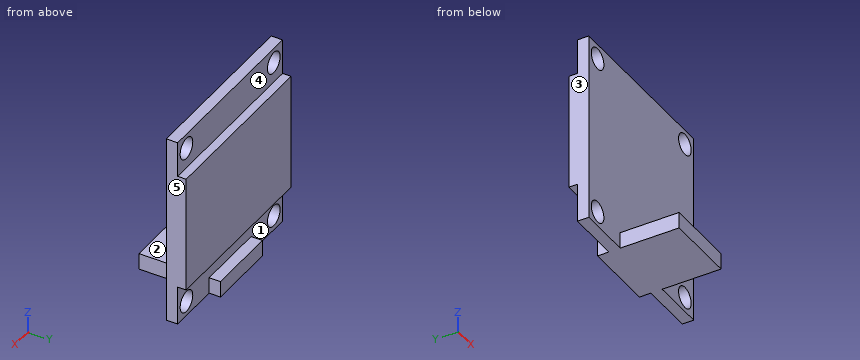
from build123d import *

# Parameters (mm, degrees)
SKETCH_1_W           = 25
SKETCH_1_H           = 27
EXTRUDE_1_DEPTH      = 1.6
SKETCH_2_W           = 25
SKETCH_2_H           = 16.5
EXTRUDE_2_DEPTH      = 1.2
SKETCH_3_R           = 1.5
CUT_EXTRUDE_1_DEPTH  = 37.83150825
EXTRUDE_4_DEPTH      = 1.6
EXTRUDE_4_DEPTH_BACK = 9.9
SKETCH_5_W           = 10
SKETCH_5_H           = 2.3


with BuildPart() as part:
    # 草图1 → 凸台-拉伸1 (new body)
    with BuildSketch(Plane(origin=(0, 0, 0), x_dir=(1, 0, 0), z_dir=(0, 1, 0))):
        with Locations((12.5, 13.5)):
            Rectangle(SKETCH_1_W, SKETCH_1_H)
    extrude(amount=EXTRUDE_1_DEPTH)

    # 草图2 → 凸台-拉伸2 (add)
    with BuildSketch(Plane(origin=(0, 1.6, 0), x_dir=(1, 0, 0), z_dir=(0, 1, 0))):
        with Locations((12.5, 13.25)):
            Rectangle(SKETCH_2_W, SKETCH_2_H)
    extrude(amount=EXTRUDE_2_DEPTH)

    # 草图3 → 切除-拉伸1 (cut, through all)
    with BuildSketch(Plane(origin=(0, 1.6, 0), x_dir=(1, 0, 0), z_dir=(0, 1, 0))):
        with Locations(Location((2.1, 24.9, 0), (0, 0, 270))):
            Circle(SKETCH_3_R)
        with Locations(Location((22.9, 24.9, 0), (0, 0, 90))):
            Circle(SKETCH_3_R)
        with Locations(Location((22.9, 2.1, 0), (0, 0, 270))):
            Circle(SKETCH_3_R)
        with Locations(Location((2.1, 2.1, 0), (0, 0, 90))):
            Circle(SKETCH_3_R)
    extrude(amount=-CUT_EXTRUDE_1_DEPTH, mode=Mode.SUBTRACT)

    # 草图5 → 凸台-拉伸4 (add, two sides: drawn at the far end of the back side and taken through both)
    with BuildSketch(Plane(origin=(0, 1.6, 0), x_dir=(1, 0, 0), z_dir=(0, 1, 0)).offset(-EXTRUDE_4_DEPTH_BACK)):
        with Locations((12.5, 25.85)):
            Rectangle(SKETCH_5_W, SKETCH_5_H)
    extrude(amount=EXTRUDE_4_DEPTH + EXTRUDE_4_DEPTH_BACK)


solid = part.part
Source: CAD feature listing. Evaluate the final solid. Frame: model axes, mm. Face numbers are marked on the shaded views. A direction names the side the tool comes from. Coordinates: 2 decimals unless noted, no trailing zeros. Write each loop counter-clockwise with the first axis right and the second up, starting at its lowest first coordinate (ties: lowest second). Pieces come first, ordered by that corner, then holes. Notation, with made-up numbers: M 72.5,26.25 L 127.5,26.25 A3 ccw 127.5,30.25 Z; hole C 55,55.25 d9. An arc over 180 degrees is marked long. Use a Markdown table: item, result.
1) Ray query, L1, parallel to X at y = 1.15, z = -2.1; L2, parallel to Z at x = 13.75, y = -7.5; L3, parallel to Y at x = 18.75, z = -12.75. Return the intervals inside material, ascending.
Conclusion:
| item | result |
|---|---|
| L1 | x = 0 to 0.6, 3.6 to 21.4, 24.4 to 25 |
| L2 | z = -27 to -24.7 |
| L3 | y = 0 to 2.8 |
2) Section C-C, the plane x = 5.5. Output: boundary loops of the cut face in (y, z).
Conclusion:
| item | result |
|---|---|
| outline | M 0,-27 L 1.6,-27 L 1.6,-21.5 L 2.8,-21.5 L 2.8,-5 L 1.6,-5 L 1.6,0 L 0,0 Z |
3) Section A-A, the plane z = -2.1. Output: boundary loops of the cut face in (x, y), then the cut area to 3 significant figures.
Conclusion:
| item | result |
|---|---|
| outline | M 0,0 L 0.6,0 L 0.6,1.6 L 0,1.6 Z; M 3.6,0 L 21.4,0 L 21.4,1.6 L 3.6,1.6 Z; M 24.4,0 L 25,0 L 25,1.6 L 24.4,1.6 Z |
| area | 30.4 mm^2 |
4) First-contact query: pin 1 Ø5 at (x, z) = (14.5, -10.5) entering from +Y; pin 2 Ø1.3 at (x, y) = (18, 2.5) entering from +Z; pin 3 Ø4 at (x, z) = (22.9, -24.9) entering from -Y; pin 4 Ø2.5 at (x, z) = (2.1, -2.1) entering from +Y. Flat tips, straight axial feed; report the tip coordinate or a pass-through.
Conclusion:
| item | result |
|---|---|
| pin 1 | stops at y = 2.8 |
| pin 2 | stops at z = -5 |
| pin 3 | stops at y = 0 |
| pin 4 | passes through |
5) Section D-D, the plane y = -2.25. Output: boundary loops of the cut face in (x, z).
Conclusion:
| item | result |
|---|---|
| outline | M 7.5,-27 L 17.5,-27 L 17.5,-24.7 L 7.5,-24.7 Z |
6) Section B-B, the plane x = 2.1. Output: boundary loops of the cut face in (y, z).
Conclusion:
| item | result |
|---|---|
| outline | M 0,-27 L 1.6,-27 L 1.6,-26.4 L 0,-26.4 Z; M 0,-23.4 L 1.6,-23.4 L 1.6,-21.5 L 2.8,-21.5 L 2.8,-5 L 1.6,-5 L 1.6,-3.6 L 0,-3.6 Z; M 0,-0.6 L 1.6,-0.6 L 1.6,0 L 0,0 Z |
7) Mould query, pull axis Z, two halves, no side actions, for the marked faces 1, 2 and 3. Classes: pulls with the +Z half, pulls with the -Z half, needs draft (parallel to the pull), parting line crosses it, or undercut.
Conclusion:
| item | result |
|---|---|
| face 1 | undercut |
| face 2 | pulls with the +Z half |
| face 3 | needs draft |
8) Reachability of the marked faces 4 and 5 from +Z, -Z, +X, -X, +Y, -Y: full face, straight path, thin tool, end or side. Return the list, or none.
Conclusion:
| item | result |
|---|---|
| face 4 | +Z, +X, -X, +Y |
| face 5 | +Z, -Z, +X, +Y, -Y |
